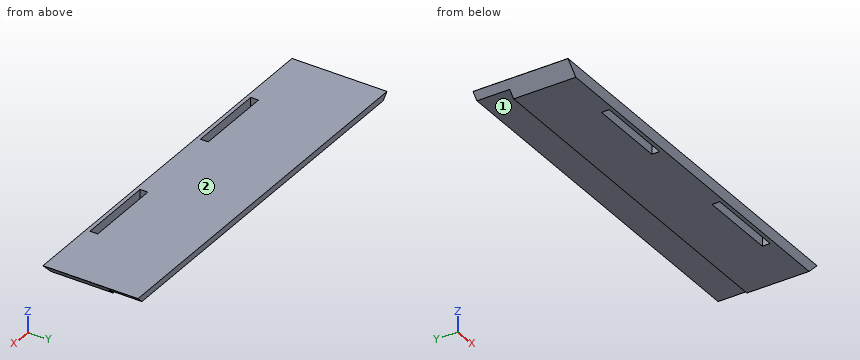
Autodesk Inventor part; units mm, degrees
ref_plane "YZ Plane" through (0, 0, 0) normal (1, 0, 0) x (0, 1, 0)
ref_plane "XZ Plane" through (0, 0, 0) normal (0, 1, 0) x (-1, 0, 0)
ref_plane "XY Plane" through (0, 0, 0) normal (0, 0, 1) x (1, 0, 0)
sketch "Sketch1" plane through (0, 0, 0) normal (1, 0, 0) x (0, 1, 0)
  line L0 (0, 0) -> (155.1, 0)
  line L1 (155.1, 0) -> (155.1, -10)
  line L2 (0, -20) -> (0, 0)
  line L3 (155.1, -10) -> (101.6, -10)
  line L4 (101.6, -10) -> (101.6, -20)
  line L5 (101.6, -20) -> (0, -20)
  dimension "d0" = 53.5
  dimension "d1" = 155.1
  dimension "d2" = 10
  dimension "d3" = 10
  dimension "d4" = 20
extrude "Extrusion1" add sketch "Sketch1" along normal blind 629.2342
chamfer "Chamfer1" distance 19.812 angle 45 1 edges at (629.2342, 50.8, -20)
chamfer "Chamfer2" distance 19.812 angle 45 1 edges at (0, 50.8, -20)
sketch "Sketch2" plane through (609.4222, 0, -20) normal (0, 0, -1) x (-1, 0, 0)
  line L0 (589.6102, 0) -> (0, 0)
  line L1 (0, 0) -> (0, 6.35)
  line L2 (0, 0) -> (0, 101.6)
  line L3 (0, 6.35) -> (88.9, 6.35)
  line L4 (88.9, 6.35) -> (88.9, 26.35)
  line L5 (88.9, 26.35) -> (215.9, 26.35)
  line L6 (215.9, 26.35) -> (215.9, 6.35)
  line L7 (215.9, 6.35) -> (368.3, 6.35)
  line L8 (368.3, 6.35) -> (368.3, 19.05)
  line L9 (368.3, 19.05) -> (495.3, 19.05)
  line L10 (495.3, 19.05) -> (495.3, 6.35)
  line L11 (495.3, 6.35) -> (589.6102, 6.35)
  line L12 (589.6102, 101.6) -> (589.6102, 0)
  line L13 (88.9, 6.35) -> (215.9, 6.35)
  line L14 (368.3, 6.35) -> (495.3, 6.35)
  point P0 (609.4222, 0)
  dimension "d13" = 6.35
  dimension "d15" = 88.9
  dimension "d16" = 127
  dimension "d17" = 152.4
  dimension "d18" = 127
  dimension "d20" = 20
  dimension "d21" = 20
  dimension "d22" = 12.7
  dimension "d23" = 12.7
sketch "Sketch3" plane through (609.4222, 0, -20) normal (0, 0, -1) x (-1, 0, 0)
  line L0 (589.6102, 0) -> (0, 0)
  line L1 (0, 0) -> (0, 6.35)
  line L2 (0, 0) -> (0, 101.6)
  line L3 (0, 6.35) -> (88.9, 6.35)
  line L4 (88.9, 6.35) -> (88.9, 19.05)
  line L5 (88.9, 19.05) -> (215.9, 19.05)
  line L6 (215.9, 19.05) -> (215.9, 6.35)
  line L7 (215.9, 6.35) -> (368.3, 6.35)
  line L8 (368.3, 6.35) -> (368.3, 26.35)
  line L9 (368.3, 26.35) -> (495.3, 26.35)
  line L10 (495.3, 26.35) -> (495.3, 6.35)
  line L11 (495.3, 6.35) -> (589.6102, 6.35)
  line L12 (589.6102, 101.6) -> (589.6102, 0)
  line L13 (88.9, 6.35) -> (215.9, 6.35)
  line L14 (368.3, 6.35) -> (495.3, 6.35)
  line L15 (-19.812, 0) -> (0, 0)
  line L16 (0, 6.35) -> (0, 0)
  point P0 (609.4222, 0)
  point P1 (609.4222, 0)
  dimension "d24" = 6.35
  dimension "d25" = 88.9
  dimension "d26" = 127
  dimension "d27" = 152.4
  dimension "d28" = 127
  dimension "d29" = 12.7
  dimension "d30" = 12.7
  dimension "d31" = 20
  dimension "d32" = 20
  dimension "d37" = 6.35
extrude "Extrusion2" cut sketch "Sketch3" against normal blind 508 contours L4 L5 L6 L13
extrude "Extrusion3" cut sketch "Sketch2" against normal blind 508 contours L14 L8 L9 L10
properties part number "SkinnySideWidth" material "Wood (Birch)"
The model under review builds one solid part; all positions refer to its coordinate system, in mm. Face numbers are marked on the shaded views. A direction names the side the tool comes from. Give positions to 0.01 mm unless a question says otherwise; leave off trailing zeros. Write each loop counter-clockwise with the first axis right and the second up, starting at its lowest first coordinate (ties: lowest second). Pieces come first, ordered by that corner, then holes. Notation, with made-up numbers: M -8.75,60 L 41.25,60 A26 cw 41.25,85 Z; hole C 10,27.25 d1. An arc over 180 degrees is marked long. One line per question, with ' | ' between items. Start each with the question number.
Item 1: We need section A-A on x = 162. Write out the cut boundary in (y, z), plus the area to 3 significant figures.
Item 2: We need section D-D on x = 350. Write out the cut boundary in (y, z).
Item 3: For pin 1 (1.5 mm diameter, centred on x = 72, y = 126.5, fed in from -Z); pin 2 (5 mm diameter, centred on x = 399, z = -15, fed in from +Y); pin 3 (1 mm diameter, centred on y = 105, z = -3.5, fed in from +X), all flat-tipped, find the tip position at first contact; note any pin that passes through.
Item 4: We need section B-B on y = 140.5. Write out the cut boundary in (x, z), plus the area to 3 significant figures.
Item 5: We need section C-C on z = -14.75. Write out the cut boundary in (x, y), plus the area to 3 significant figures.
Item 6: Wall thickness on line 1 (Y direction, x = 148.5, z = -7.25); line 2 (Y direction, x = 498, z = -11.25); line 3 (Z direction, x = 430.5, y = 119.5): over which ranges is each line inside the solid? List them lowest first. Write a range as from..to.
Item 7: For the marked faces 1 and 2, list the 3-axis set-ups (+Z, -Z, +X, -X, +Y, -Y) from which the entire face can be reached by the end or side of a thin tool; tool diameter is ignored.
Results found:
1) outline: M 0,-20 L 6.35,-20 L 6.35,0 L 0,0 Z; M 19.05,-20 L 101.6,-20 L 101.6,-10 L 155.1,-10 L 155.1,0 L 19.05,0 Z | area: 2,310 mm2
2) outline: M 0,-20 L 101.6,-20 L 101.6,-10 L 155.1,-10 L 155.1,0 L 0,0 Z
3) pin 1: stops at z = -10 | pin 2: stops at y = 101.6 | pin 3: stops at x = 626.42
4) outline: M 0,-0.19 L 9.81,-10 L 619.42,-10 L 629.23,-0.19 L 629.23,0 L 0,0 Z | area: 6,200 mm2
5) outline: M 14.56,0 L 614.67,0 L 614.67,101.6 L 14.56,101.6 Z; hole M 114.12,6.35 L 241.12,6.35 L 241.12,19.05 L 114.12,19.05 Z; hole M 393.52,6.35 L 520.52,6.35 L 520.52,19.05 L 393.52,19.05 Z | area: 57,700 mm2
6) line 1: y = 0..6.35, 19.05..155.1 | line 2: y = 0..6.35, 19.05..101.6 | line 3: z = -10..0
7) face 1: -Z, +X, -X, +Y | face 2: +Z, +X, -X, +Y, -Y
